Source: CAD feature listing. Evaluate the final solid. Frame: model axes, mm. A direction names the side the tool comes from. Coordinates: 2 decimals unless noted, no trailing zeros. Order: outer loops, then holes, each group sorted by start corner. A loop starts at its lowest first (then second) coordinate and runs counter-clockwise, first axis right, second up. Notation, with made-up numbers: (-23.75, -32.5) -> (-4.75, -32.5) arc R22 cw to (-4.75, -2.5) -> close; hole circle Ø4 at (21.25, 83.25). An arc over 180 degrees is marked (long way). Put each result on its own line as item: value.
Autodesk Inventor part; units mm, degrees
ref_plane "YZ Plane" through (0, 0, 0) normal (1, 0, 0) x (0, 1, 0)
ref_plane "XZ Plane" through (0, 0, 0) normal (0, 1, 0) x (-1, 0, 0)
ref_plane "XY Plane" through (0, 0, 0) normal (0, 0, 1) x (1, 0, 0)
sketch "Sketch1" plane through (0, 0, 0) normal (1, 0, 0) x (0, 1, 0)
  line L0 (0, 0) -> (10, 0)
  line L1 (10, 1600) -> (0, 1600)
  line L2 (0, 1600) -> (0, 10)
  line L3 (10, 100) -> (560, 100)
  line L4 (570, 100) -> (570, 90)
  line L5 (560, 90) -> (10, 90)
  line L6 (570, 0) -> (560, 0)
  line L7 (560, 1600) -> (570, 1600)
  line L8 (570, 1600) -> (570, 10)
  line L9 (10, 600) -> (560, 600)
  line L10 (10, 590) -> (560, 590)
  line L11 (10, 1100) -> (560, 1100)
  line L12 (10, 1090) -> (560, 1090)
  line L13 (540, 0) -> (590, 0)
  line L14 (590, 0) -> (590, 10)
  line L15 (540, 10) -> (540, 0)
  line L16 (-20, 0) -> (30, 0)
  line L17 (30, 0) -> (30, 10)
  line L18 (-20, 10) -> (-20, 0)
  line L19 (30, 10) -> (10, 10)
  line L20 (0, 10) -> (-20, 10)
  line L21 (590, 10) -> (570, 10)
  line L22 (560, 10) -> (540, 10)
  line L23 (560, 10) -> (560, 90)
  line L24 (10, 10) -> (10, 90)
  line L25 (10, 100) -> (10, 590)
  line L26 (560, 100) -> (560, 590)
  line L27 (560, 600) -> (560, 1090)
  line L28 (560, 1100) -> (560, 1600)
  line L29 (10, 600) -> (10, 1090)
  line L30 (10, 1100) -> (10, 1600)
  dimension "d0" = 10
  dimension "d1" = 1600
  dimension "d2" = 560
  dimension "d3" = 10
  dimension "d4" = 10
  dimension "d5" = 1600
  dimension "d6" = 50
  dimension "d7" = 10
  dimension "d8" = 50
  dimension "d9" = 10
extrude "Extrusion1" add sketch "Sketch1" along normal blind 300
sketch "Sketch2" plane through (0, 10, 1600) normal (0, 1, 0) x (1, 0, 0)
  line L0 (0, 500) -> (200, 500)
  line L1 (200, 500) -> (200, 100)
  line L2 (200, 100) -> (0, 100)
  line L3 (0, 100) -> (0, 500)
  line L4 (200, 100) -> (180, 100)
  line L5 (180, 100) -> (180, 165)
  line L6 (180, 165) -> (200, 165)
  line L7 (200, 165) -> (200, 100)
  line L8 (180, 100) -> (0, 100)
  line L9 (0, 100) -> (0, 150)
  line L10 (0, 150) -> (180, 150)
  line L11 (180, 150) -> (180, 100)
  line L12 (180, 150) -> (170, 150)
  line L13 (170, 150) -> (170, 200)
  line L14 (170, 200) -> (180, 200)
  line L15 (180, 200) -> (180, 150)
  line L16 (0, 1000) -> (0, 510)
  line L17 (0, 1000) -> (180, 1000)
  line L18 (180, 1000) -> (180, 650)
  line L19 (180, 650) -> (0, 650)
  line L20 (0, 650) -> (0, 1000)
  line L21 (0, 1500) -> (180, 1500)
  line L22 (180, 1500) -> (180, 1150)
  line L23 (180, 1150) -> (0, 1150)
  line L24 (0, 1150) -> (0, 1500)
  line L25 (180, 650) -> (170, 650)
  line L26 (170, 650) -> (170, 700)
  line L27 (170, 700) -> (180, 700)
  line L28 (180, 700) -> (180, 650)
  line L29 (180, 1150) -> (170, 1150)
  line L30 (170, 1150) -> (170, 1200)
  line L31 (170, 1200) -> (180, 1200)
  line L32 (180, 1200) -> (180, 1150)
  point P0 (0, 1600)
  dimension "d12" = 200
  dimension "d13" = 400
  dimension "d14" = 20
  dimension "d15" = 65
  dimension "d16" = 180
  dimension "d17" = 50
  dimension "d18" = 10
  dimension "d19" = 50
  dimension "d20" = 180
  dimension "d21" = 350
  dimension "d22" = 180
  dimension "d23" = 350
  dimension "d24" = 10
  dimension "d25" = 50
  dimension "d26" = 10
  dimension "d27" = 50
extrude "Extrusion2" add sketch "Sketch2" along normal blind 550 contours L13 L14 L15 L5 L10 | L26 L27 L18 L19 | L22 L23 L30 L31
properties part number "MoldStore"
1. Cut plane C-C on x = 54.5. Output: boundary loops of the cut face in (y, z), plus the area to 3 significant figures.
Numbers:
outline: (-20, 0) -> (30, 0) -> (30, 10) -> (10, 10) -> (10, 90) -> (560, 90) -> (560, 10) -> (540, 10) -> (540, 0) -> (590, 0) -> (590, 10) -> (570, 10) -> (570, 1600) -> (560, 1600) -> (560, 1100) -> (10, 1100) -> (10, 1600) -> (0, 1600) -> (0, 10) -> (-20, 10) -> close; hole (10, 100) -> (560, 100) -> (560, 590) -> (10, 590) -> close; hole (10, 600) -> (560, 600) -> (560, 1090) -> (10, 1090) -> close
area: 49,300 mm2
2. Ray query, line 1 along Z through (x, y) = (258.5, 461.5); line 2 along Z through (x, y) = (174, 272); line 3 along Z through (x, y) = (86, 545). Return the intervals inside material, ascending.
Numbers:
line 1: z = 90 to 100, 590 to 600, 1090 to 1100
line 2: z = 90 to 100, 400 to 450, 590 to 600, 900 to 950, 1090 to 1100, 1400 to 1450
line 3: z = 0 to 10, 90 to 100, 590 to 600, 1090 to 1100
3. Cut plane A-A on y = 373.5. Output: boundary loops of the cut face in (x, z), plus the area to 3 significant figures.
Numbers:
outline: (0, 90) -> (300, 90) -> (300, 100) -> (0, 100) -> close; (0, 590) -> (300, 590) -> (300, 600) -> (0, 600) -> close; (0, 1090) -> (300, 1090) -> (300, 1100) -> (0, 1100) -> close; (170, 400) -> (180, 400) -> (180, 450) -> (170, 450) -> close; (170, 900) -> (180, 900) -> (180, 950) -> (170, 950) -> close; (170, 1400) -> (180, 1400) -> (180, 1450) -> (170, 1450) -> close
area: 10,500 mm2
4. Set-up query: faces 1 (the flat face through (148, 560, 49)), 2 (the flat face through (180, 281, 1425)), 3 (the flat face through (180, 281, 425)). Return all of +Z, -Z, +X, -X, +Y, -Y with unobstructed straight access to the full face (end or side cutting, diameter ignored); none if empty.
Numbers:
face 1: +X, -X
face 2: +Z, +X
face 3: +X
5. Cut plane B-B on z = 819.5. Output: boundary loops of the cut face in (x, y).
Numbers:
outline: (0, 0) -> (300, 0) -> (300, 10) -> (0, 10) -> close; (0, 560) -> (300, 560) -> (300, 570) -> (0, 570) -> close
6. First-contact query: pin 1 (16 mm diameter, centred on x = 182.5, y = 547, fed in from +Z); pin 2 (5 mm diameter, centred on x = 89, y = 372, fed in from -Z); pin 3 (4 mm diameter, centred on x = 255, z = 361.5, fed in from -Y). Flat tips, straight axial feed; report the tip coordinate or a pass-through.
Numbers:
pin 1: stops at z = 1450
pin 2: stops at z = 90
pin 3: stops at y = 0
7. Pull-direction query (Y, two-part tool) for faces 4 (the flat face through (148, 0, 816)), 5 (the flat face through (0, 284, 93)), 6 (the flat face through (148, 10, 1346)); classes: pulls with the +Y half, pulls with the -Y half, needs draft (parallel to the pull), parting line crosses it, or undercut.
Numbers:
face 4: pulls with the -Y half
face 5: needs draft
face 6: undercut
